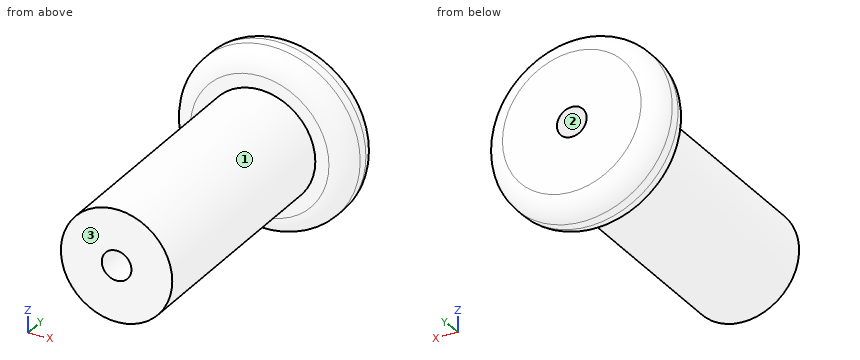
```python
from build123d import *

# Parameters (mm, degrees)
F0_R     = 22.86
F0_R_2   = 14.2875
F2_DEPTH = 12.7
F3_R     = 5.08
F0_R_3   = 3.81
F5_DEPTH = 76.2


# Not quite as in the source:
# - the program builds the solid bodies; features that only make, move or delete a surface that nothing else refers to are left out


with BuildPart() as f2:
    # F0 (on Front) → F2 (new body)
    with BuildSketch(Plane.XZ):
        Circle(F0_R)
        Circle(F0_R_2, mode=Mode.SUBTRACT)
    extrude(amount=F2_DEPTH)

    # F3
    f3_edges = [f2.edges().sort_by_distance(p)[0] for p in [
        (-22.86, 0, 0),
        (-22.86, -12.7, 0),
    ]]
    fillet(f3_edges, radius=F3_R)

    # F0 (on Front) → F5 (join)
    with BuildSketch(Plane.XZ):
        Circle(F0_R_2)
        Circle(F0_R_3, mode=Mode.SUBTRACT)
    extrude(amount=F5_DEPTH)


solid = f2.part
```
Here's how the part is built. I have some questions about the finished solid (model axes, mm). Face numbers are marked on the shaded views. Coordinates: 2 decimals unless noted, no trailing zeros. Order: outer loops, then holes, each group sorted by start corner. A loop starts at its lowest first (then second) coordinate and runs counter-clockwise, first axis right, second up. Notation, with made-up numbers: (11, 35.5) - (16, 35.5) arc R8 cw to (16, 40.5) - close; hole circle Ø6 at (-11.5, -22). An arc over 180 degrees is marked (long way). One line per question, with ' | ' between items.
(1) Suppose I cut it at A-A on z = 0. List the corners of the cut face in (x, y) for me.
Report:
outline: (-22.86, -7.62) arc R5.08 ccw to (-17.78, -12.7) - (-14.29, -12.7) - (-14.29, -76.2) - (-3.81, -76.2) - (-3.81, 0) - (-17.78, 0) arc R5.08 ccw to (-22.86, -5.08) - close; (3.81, -76.2) - (14.29, -76.2) - (14.29, -12.7) - (17.78, -12.7) arc R5.08 ccw to (22.86, -7.62) - (22.86, -5.08) arc R5.08 ccw to (17.78, 0) - (3.81, 0) - close
(2) Suppose I cut it at D-D on y = -11.5. List the corners of the cut face in (x, z) for me, and give its area (3 significant figures).
Report:
outline: circle Ø42.12 at (0, 0); hole circle Ø7.62 at (0, 0) | area: 1,350 mm2
(3) If we mould it in two halves opening along Z, with no side actions, what happens to the marked faces 1, 2 and 3? For each: pulls with the +Z half, pulls with the -Z half, needs draft (parallel to the pull), parting line crosses it, or undercut.
Report:
face 1: parting line crosses it | face 2: undercut | face 3: needs draft
(4) Suppose I cut it at B-B on x = 0. List the corners of the cut face in (y, z) for me, and give its area (3 significant figures).
Report:
outline: (-76.2, -14.29) - (-12.7, -14.29) - (-12.7, -17.78) arc R5.08 ccw to (-7.62, -22.86) - (-5.08, -22.86) arc R5.08 ccw to (0, -17.78) - (0, -3.81) - (-76.2, -3.81) - close; (-76.2, 3.81) - (0, 3.81) - (0, 17.78) arc R5.08 ccw to (-5.08, 22.86) - (-7.62, 22.86) arc R5.08 ccw to (-12.7, 17.78) - (-12.7, 14.29) - (-76.2, 14.29) - close | area: 1,790 mm2
(5) Will these pins go through, and if not, where does the flat tip stop? pin 1 (3 mm diameter, centred on x = -17, z = -1, fed in from +Y); pin 2 (6 mm diameter, centred on x = 0, z = 0, fed in from +Y); pin 3 (8 mm diameter, centred on x = 0, y = -36, fed in from +Z); pin 4 (1 mm diameter, centred on x = 6.5, y = -58.5, fed in from +Z).
Report:
pin 1: stops at y = 0 | pin 2: passes through | pin 3: stops at z = 14.29 | pin 4: stops at z = 12.97
(6) If I drill on L1, parallel to Z at x = 0, y = -38; L2, parallel to Z at x = -3.5, y = -53.5; L3, parallel to X at y = -2.5, z = -2.5, over which ranges is the centre line in solid material (lowest first)?
Report:
L1: z = -14.29 to -3.81, 3.81 to 14.29 | L2: z = -13.85 to -1.51, 1.51 to 13.85 | L3: x = -22.01 to -2.88, 2.88 to 22.01
(7) Suppose I cut it at C-C on y = -48.5. List the corners of the cut face in (x, z) for me (1 decimal), and give its area (3 significant figures).
Report:
outline: circle Ø28.6 at (0, 0); hole circle Ø7.6 at (0, 0) | area: 596 mm2
